```python
from build123d import *

# Parameters (mm, degrees)
BODY_DEPTH              = 35
SKETCH3_R               = 7.5
SHAFT_HOLE_DEPTH        = 40
SKETCH4_R               = 2.5
BOSS_EXTRUDE1_DEPTH     = 5
SKETCH5_R               = 10
BEARING_DEPTH           = 5
MIRROR5_COPY_1_SKETCH_R = 10
MIRROR5_COPY_1_DEPTH    = 5
SKETCH6_R               = 2.5
CUT_EXTRUDE1_DEPTH      = 55.224072145


with BuildPart() as part:
    # Sketch1 → body (new body)
    with BuildSketch(Plane(origin=(0, 0, 0), x_dir=(0, 0, -1), z_dir=(1, 0, 0))):
        with BuildLine():
            Line((-15, -15), (-15, -25))
            Line((-15, -25), (0, -25))
            Line((0, -25), (0, 25))
            Line((0, 25), (-15, 25))
            Line((-15, 25), (-15, 15))
            ThreePointArc((-15, 15), (-30, 0), (-15, -15))
        make_face()
    extrude(amount=BODY_DEPTH)

    # Sketch3 → shaft hole (cut)
    with BuildSketch(Plane(origin=(35, 0, 0), x_dir=(0, 0, -1), z_dir=(1, 0, 0))):
        with Locations((-15, 0)):
            Circle(SKETCH3_R)
    extrude(amount=-SHAFT_HOLE_DEPTH, mode=Mode.SUBTRACT)

    # Sketch4 → Boss-Extrude1 (add)
    with BuildSketch(Plane(origin=(0, 25, 0), x_dir=(1, 0, 0), z_dir=(0, 1, 0))):
        with Locations(Location((4.5, -5, 0), (0, 0, 90))):
            Circle(SKETCH4_R)
        with Locations(Location((30.5, -5, 0), (0, 0, 90))):
            Circle(SKETCH4_R)
    boss_extrude1 = extrude(amount=BOSS_EXTRUDE1_DEPTH)

    # Mirror1: Boss-Extrude1 across plane
    add(boss_extrude1.mirror(Plane.ZX))

    # Sketch5 → bearing (add)
    with BuildSketch(Plane(origin=(0, 30, 0), x_dir=(1, 0, 0), z_dir=(0, 1, 0))):
        with Locations(Location((4.5, -5, 0), (0, 0, 270))):
            Circle(SKETCH5_R)
    bearing = extrude(amount=-BEARING_DEPTH)

    # Mirror2: bearing across plane
    add(bearing.mirror(Plane.ZX))

    # Mirror5: bearing across plane
    add(bearing.mirror(Plane(origin=(17.5, 0, 0), x_dir=(0, 0, 1), z_dir=(1, 0, 0))))

    # Mirror5 copy 1 sketch → Mirror5 copy 1 (add)
    with BuildSketch(Plane(origin=(35, -30, 0), x_dir=(-1, 0, 0), z_dir=(0, -1, 0))):
        with Locations(Location((4.5, -5, 0), (0, 0, 270))):
            Circle(MIRROR5_COPY_1_SKETCH_R)
    extrude(amount=-MIRROR5_COPY_1_DEPTH)

    # Sketch6 → Cut-Extrude1 (cut, through all)
    with BuildSketch(Plane.XY.offset(15)):
        with Locations((5, 20)):
            Circle(SKETCH6_R)
        with Locations((30, 20)):
            Circle(SKETCH6_R)
        with Locations((30, -20)):
            Circle(SKETCH6_R)
        with Locations((5, -20)):
            Circle(SKETCH6_R)
    extrude(amount=-CUT_EXTRUDE1_DEPTH, mode=Mode.SUBTRACT)


solid = part.part
```
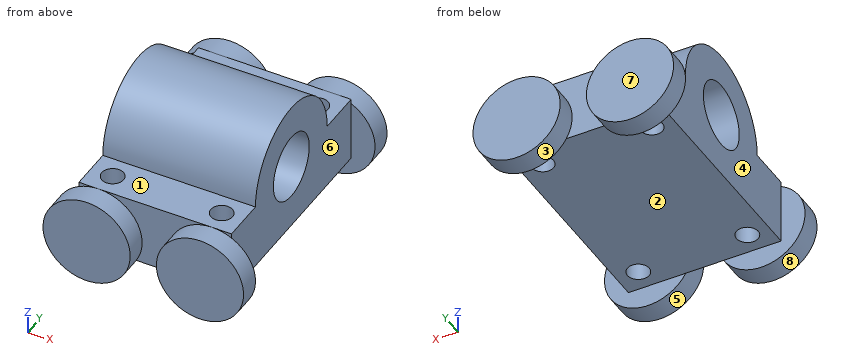
Check sheet for the modelled part. Datum: model origin and axes. Units: mm. Face numbers are marked on the shaded views. A direction names the side the tool comes from. Coordinates: 2 decimals unless noted, no trailing zeros. Loops run counter-clockwise (first coordinate to the right, second up) from the corner with the lowest first, then second, coordinate; pieces in that order, holes last.
1) Access from +Z, -Z, +X, -X, +Y, -Y to the whole of each face (thin tool, end or side, straight path). Record for the marked faces 1, 2, 3, 4 and 5.
2) Sectioned sample at A-A (z = 9). Record the boundary of the cut face in (x, y).
3) Material ranges on probe 1 along Y at (x, z) = (5, 5.5); probe 2 along Y at (x, z) = (30, 8.5); probe 3 along Y at (x, z) = (28, 10.5), recorded low to high.
4) Sectioned sample at C-C (z = 5). Record the boundary of the cut face in (x, y), and give its area (3 significant figures).
5) Sectioned sample at D-D (x = -2.5). Record the boundary of the cut face in (y, z), and give its area (3 significant figures).
6) Release check for a two-part mould opening along X. For the marked faces 6, 7 and 8 record: released by +X, released by -X, zero draft, split by the parting line, or undercut.
7) Gauge pin test, flat ends, axial feed: pin 1 (6.5 mm diameter, centred on x = 30, y = 20, fed in from -Z); pin 2 (12 mm diameter, centred on y = 19.5, z = 19.5, fed in from -X); pin 3 (8 mm diameter, centred on x = 11, y = -8.5, fed in from +Z); pin 4 (9 mm diameter, centred on y = 0, z = 15, fed in from +X). Record the tip position at first contact, or that the pin passes through.
8) Sectioned sample at B-B (y = 0). Record the boundary of the cut face in (x, z), and give its area (3 significant figures).
Check sheet entries:
1. face 1: +Z, +X, -X, -Y
1. face 2: -Z, +X, -X
1. face 3: +Y
1. face 4: +Z, -Z, -X
1. face 5: -Y
2. outline: (-4.67, -30) - (13.67, -30) - (13.67, -25) - (21.33, -25) - (21.33, -30) - (39.67, -30) - (39.67, -25) - (35, -25) - (35, -4.5) - (0, -4.5) - (0, -25) - (-4.67, -25) - close; (-4.67, 25) - (0, 25) - (0, 4.5) - (35, 4.5) - (35, 25) - (39.67, 25) - (39.67, 30) - (21.33, 30) - (21.33, 25) - (13.67, 25) - (13.67, 30) - (-4.67, 30) - close; hole circle Ø5 at (5, -20); hole circle Ø5 at (5, 20); hole circle Ø5 at (30, -20); hole circle Ø5 at (30, 20)
3. probe 1: y = -30 to -22.5, -17.5 to 17.5, 22.5 to 30
3. probe 2: y = -30 to -22.5, -17.5 to -3.74, 3.74 to 17.5, 22.5 to 30
3. probe 3: y = -30 to -21.5, -18.5 to -6, 6 to 18.5, 21.5 to 30
4. outline: (-5.5, -30) - (14.5, -30) - (14.5, -25) - (20.5, -25) - (20.5, -30) - (40.5, -30) - (40.5, -25) - (35, -25) - (35, 25) - (40.5, 25) - (40.5, 30) - (20.5, 30) - (20.5, 25) - (14.5, 25) - (14.5, 30) - (-5.5, 30) - (-5.5, 25) - (0, 25) - (0, -25) - (-5.5, -25) - close; hole circle Ø5 at (5, -20); hole circle Ø5 at (5, 20); hole circle Ø5 at (30, -20); hole circle Ø5 at (30, 20)
4. area: 2,070 mm2
5. outline: (-30, -2.14) - (-25, -2.14) - (-25, 12.14) - (-30, 12.14) - close; (25, -2.14) - (30, -2.14) - (30, 12.14) - (25, 12.14) - close
5. area: 143 mm2
6. face 6: released by +X
6. face 7: zero draft
6. face 8: undercut
7. pin 1: stops at z = 0
7. pin 2: stops at x = 0
7. pin 3: stops at z = 29.31
7. pin 4: passes through
8. outline: (0, 0) - (35, 0) - (35, 7.5) - (0, 7.5) - close; (0, 22.5) - (35, 22.5) - (35, 30) - (0, 30) - close
8. area: 525 mm2
